Source: CAD feature listing. Evaluate the final solid. Frame: model axes, mm. Round coordinates to 2 decimals unless told otherwise and drop trailing zeros. Write each loop counter-clockwise with the first axis right and the second up, starting at its lowest first coordinate (ties: lowest second). Pieces come first, ordered by that corner, then holes. Notation, with made-up numbers: M 58.25,-1.75 L 110.25,-1.75 A20 ccw 110.25,18.25 Z; hole C 70,36.5 d2. An arc over 180 degrees is marked long. Use a Markdown table: item, result.
```python
from build123d import *

# Parameters (mm, degrees)
SKETCH1_R           = 23
SKETCH1_R_2         = 3.175
BOSS_EXTRUDE1_DEPTH = 4


with BuildPart() as part:
    # Sketch1 → Boss-Extrude1 (new body)
    with BuildSketch(Plane(origin=(0, 0, 0), x_dir=(0, 0, -1), z_dir=(1, 0, 0))):
        Circle(SKETCH1_R)
        Circle(SKETCH1_R_2, mode=Mode.SUBTRACT)
        with Locations((0, 18.5125)):
            Circle(SKETCH1_R_2, mode=Mode.SUBTRACT)
        with Locations((-18.5125, 0)):
            Circle(SKETCH1_R_2, mode=Mode.SUBTRACT)
        with Locations((0, -18.5125)):
            Circle(SKETCH1_R_2, mode=Mode.SUBTRACT)
        with Locations((18.5125, 0)):
            Circle(SKETCH1_R_2, mode=Mode.SUBTRACT)
        with BuildLine():
            Line((4.7625, 6.7625), (4.7625, 16.789240416))
            ThreePointArc((4.7625, 16.789240416), (5.643231296, 18.446719698), (7.509737569, 18.644405103))
            ThreePointArc((7.509737569, 18.644405103), (14.212846302, 14.212846302), (18.644405103, 7.509737569))
            ThreePointArc((18.644405103, 7.509737569), (18.446719698, 5.643231296), (16.789240416, 4.7625))
            Line((16.789240416, 4.7625), (6.7625, 4.7625))
            ThreePointArc((6.7625, 4.7625), (5.348286438, 5.348286438), (4.7625, 6.7625))
        make_face(mode=Mode.SUBTRACT)
        with BuildLine():
            Line((6.7625, -4.7625), (16.789240416, -4.7625))
            ThreePointArc((16.789240416, -4.7625), (18.446719698, -5.643231296), (18.644405103, -7.509737569))
            ThreePointArc((18.644405103, -7.509737569), (14.212846302, -14.212846302), (7.509737569, -18.644405103))
            ThreePointArc((7.509737569, -18.644405103), (5.643231296, -18.446719698), (4.7625, -16.789240416))
            Line((4.7625, -16.789240416), (4.7625, -6.7625))
            ThreePointArc((4.7625, -6.7625), (5.348286438, -5.348286438), (6.7625, -4.7625))
        make_face(mode=Mode.SUBTRACT)
        with BuildLine():
            Line((-4.7625, -6.7625), (-4.7625, -16.789240416))
            ThreePointArc((-4.7625, -16.789240416), (-5.643231296, -18.446719698), (-7.509737569, -18.644405103))
            ThreePointArc((-7.509737569, -18.644405103), (-14.212846302, -14.212846302), (-18.644405103, -7.509737569))
            ThreePointArc((-18.644405103, -7.509737569), (-18.446719698, -5.643231296), (-16.789240416, -4.7625))
            Line((-16.789240416, -4.7625), (-6.7625, -4.7625))
            ThreePointArc((-6.7625, -4.7625), (-5.348286438, -5.348286438), (-4.7625, -6.7625))
        make_face(mode=Mode.SUBTRACT)
        with BuildLine():
            Line((-6.7625, 4.7625), (-16.789240416, 4.7625))
            ThreePointArc((-16.789240416, 4.7625), (-18.446719698, 5.643231296), (-18.644405103, 7.509737569))
            ThreePointArc((-18.644405103, 7.509737569), (-14.212846302, 14.212846302), (-7.509737569, 18.644405103))
            ThreePointArc((-7.509737569, 18.644405103), (-5.643231296, 18.446719698), (-4.7625, 16.789240416))
            Line((-4.7625, 16.789240416), (-4.7625, 6.7625))
            ThreePointArc((-4.7625, 6.7625), (-5.348286438, 5.348286438), (-6.7625, 4.7625))
        make_face(mode=Mode.SUBTRACT)
    extrude(amount=BOSS_EXTRUDE1_DEPTH)


solid = part.part
```
Q1. First-contact query: pin 1 Ø2 at (x, z) = (2, -10) entering from +Y; pin 2 Ø2 at (x, y) = (2.5, 16.5) entering from +Z; pin 3 Ø1 at (x, y) = (2, 8) entering from -Z. Flat tips, straight axial feed; report the tip coordinate or a pass-through.
Results are:
| item | result |
|---|---|
| pin 1 | y = 21.17 |
| pin 2 | z = 16.99 |
| pin 3 | z = -21.74 |
Q2. Mould query, pull axis Z, two halves, no side actions, for faces 1 (the cylindrical face through (1.972, 22.804, 2.994)), 2 (the flat face through (4, 2, -3)), 3 (the cylindrical face through (2, -5.4, -5.3)), 4 (the cylindrical face through (1.97, -3.1, 0.69)). Classes: +Z half, -Z half, draft (parallel to the pull), parting line (faces both ways), or undercut.
Results are:
| item | result |
|---|---|
| face 1 | parting line |
| face 2 | draft |
| face 3 | undercut |
| face 4 | undercut |
Q3. Section D-D on y = -20. Return loops of the section in (x, z), plus the area to 3 significant figures.
Results are:
| item | result |
|---|---|
| outline | M 0,-11.36 L 4,-11.36 L 4,-2.8 L 0,-2.8 Z; M 0,2.8 L 4,2.8 L 4,11.36 L 0,11.36 Z |
| area | 68.4 mm^2 |
Q4. Section A-A on z = 0. Return loops of the section in (x, y) (1 decimal), plus the area to 3 significant figures.
Results are:
| item | result |
|---|---|
| outline | M 0,-23 L 4,-23 L 4,-21.7 L 0,-21.7 Z; M 0,-15.3 L 4,-15.3 L 4,-3.2 L 0,-3.2 Z; M 0,3.2 L 4,3.2 L 4,15.3 L 0,15.3 Z; M 0,21.7 L 4,21.7 L 4,23 L 0,23 Z |
| area | 108 mm^2 |
Q5. Line query: L1, parallel to Y at x = 2.8, z = 0 (1 decimal); L2, parallel to Y at x = 3.3, z = 2; L3, parallel to Z at x = 0.4, y = -15. Output: solid intervals per line, ascending.
Results are:
| item | result |
|---|---|
| L1 | -23 to -21.7, -15.3 to -3.2, 3.2 to 15.3, 21.7 to 23 |
| L2 | -22.91 to -20.98, -16.05 to -2.47, 2.47 to 16.05, 20.98 to 22.91 |
| L3 | -17.44 to -13.38, -4.76 to 4.76, 13.38 to 17.44 |
Q6. Section C-C on z = 10.5. Return loops of the section in (x, y).
Results are:
| item | result |
|---|---|
| outline | M 0,-20.46 L 4,-20.46 L 4,-17.14 L 0,-17.14 Z; M 0,-4.76 L 4,-4.76 L 4,4.76 L 0,4.76 Z; M 0,17.14 L 4,17.14 L 4,20.46 L 0,20.46 Z |
